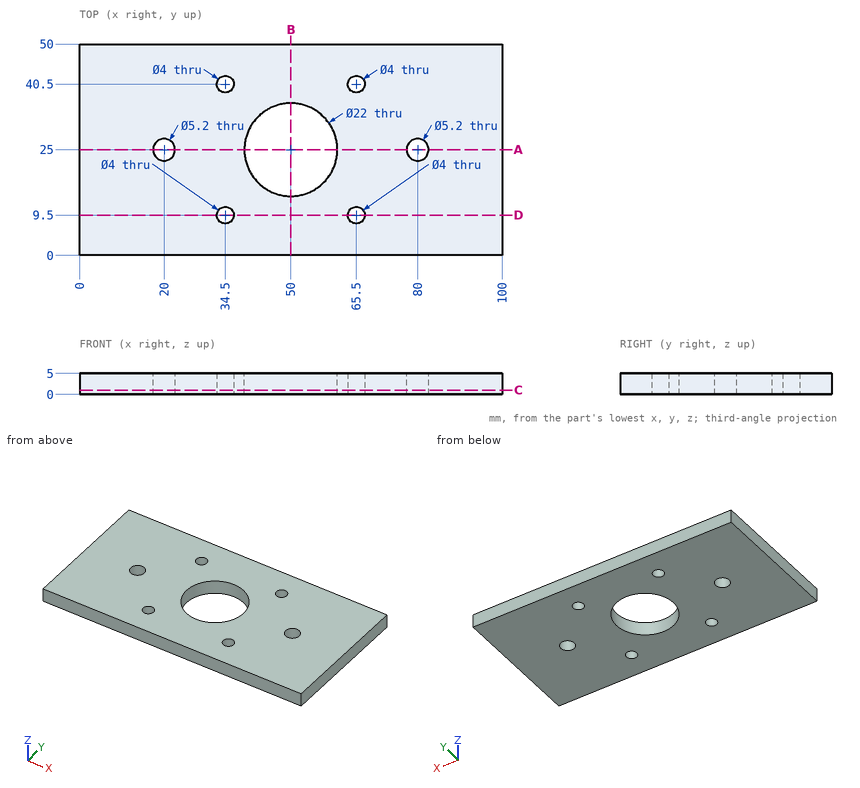
Can you work these out from the drawing? Everything is in mm from the part's minimum corner. Give positions to 0.01 mm unless a question says otherwise; leave off trailing zeros. Order: outer loops, then holes, each group sorted by start corner. A loop starts at its lowest first (then second) coordinate and runs counter-clockwise, first axis right, second up.
Item 1: If we section it at C-C, the plane z = 1: Write out the boundary of the cut face in (x, y).
Item 2: If we section it at A-A, the plane y = 25: Write out the boundary of the cut face in (x, z).
Item 3: I need wall thicknesses on line 1 (X direction, y = 25, z = 2.55); line 2 (X direction, y = 40.5, z = 4.7); line 3 (Y direction, x = 65.5, z = 2.25). Which ranges of each line are inside material? Lowest first, please.
Item 4: If we section it at B-B, the plane x = 50: Write out the boundary of the cut face in (y, z), plus the area to 3 significant figures.
Item 5: If we section it at D-D, the plane y = 9.5: Write out the boundary of the cut face in (x, z), plus the area to 3 significant figures.
Values:
1. outline: (0, 0) - (100, 0) - (100, 50) - (0, 50) - close; hole circle Ø5.2 at (20, 25); hole circle Ø4 at (34.5, 9.5); hole circle Ø4 at (34.5, 40.5); hole circle Ø22 at (50, 25); hole circle Ø4 at (65.5, 9.5); hole circle Ø4 at (65.5, 40.5); hole circle Ø5.2 at (80, 25)
2. outline: (0, 0) - (17.4, 0) - (17.4, 5) - (0, 5) - close; (22.6, 0) - (39, 0) - (39, 5) - (22.6, 5) - close; (61, 0) - (77.4, 0) - (77.4, 5) - (61, 5) - close; (82.6, 0) - (100, 0) - (100, 5) - (82.6, 5) - close
3. line 1: x = 0 to 17.4, 22.6 to 39, 61 to 77.4, 82.6 to 100
3. line 2: x = 0 to 32.5, 36.5 to 63.5, 67.5 to 100
3. line 3: y = 0 to 7.5, 11.5 to 38.5, 42.5 to 50
4. outline: (0, 0) - (14, 0) - (14, 5) - (0, 5) - close; (36, 0) - (50, 0) - (50, 5) - (36, 5) - close
4. area: 140 mm2
5. outline: (0, 0) - (32.5, 0) - (32.5, 5) - (0, 5) - close; (36.5, 0) - (63.5, 0) - (63.5, 5) - (36.5, 5) - close; (67.5, 0) - (100, 0) - (100, 5) - (67.5, 5) - close
5. area: 460 mm2
